```python
from build123d import *

# Parameters (mm, degrees)
EXTRUDE_1_DEPTH     = 15.5
SKETCH_2_R          = 4
CUT_EXTRUDE_1_DEPTH = 41.118574252
SKETCH_3_W          = 25
SKETCH_3_H          = 25.5
CUT_EXTRUDE_2_DEPTH = 43.924352063
CUT_EXTRUDE_3_REACH = 39.346
SKETCH_4_R          = 5.3
FILLET_1_R          = 1
FILLET_2_R          = 1
CHAMFER_1_SIZE      = 0.2


with BuildPart() as part:
    # ｽｹｯﾁ1 → ﾎﾞｽ - 押し出し1 (new, symmetric)
    with BuildSketch(Plane.XY):
        with BuildLine():
            Line((-18.5, 11), (-18.5, -13))
            Line((-18.5, -13), (-11.715374514, -13))
            ThreePointArc((-11.715374514, -13), (12.037359531, -12.702439747), (13.610657589, 11))
            Line((13.610657589, 11), (-18.5, 11))
        make_face()
    extrude(amount=EXTRUDE_1_DEPTH, both=True)

    # ｽｹｯﾁ2 → ｶｯﾄ - 押し出し1 (cut, through all)
    with BuildSketch(Plane.XY.offset(15.5)):
        Circle(SKETCH_2_R)
        with BuildLine():
            Line((-18.5, 2), (-14.5, 2))
            ThreePointArc((-14.5, 2), (-10.5, -2), (-14.5, -6))
            Line((-14.5, -6), (-18.5, -6))
            Line((-18.5, -6), (-18.5, 2))
        make_face()
    extrude(amount=-CUT_EXTRUDE_1_DEPTH, mode=Mode.SUBTRACT)

    # ｽｹｯﾁ3 → ｶｯﾄ - 押し出し2 (cut, through all)
    with BuildSketch(Plane.ZY.offset(18.5)):
        with Locations((0, -4.75)):
            Rectangle(SKETCH_3_W, SKETCH_3_H)
    extrude(amount=-CUT_EXTRUDE_2_DEPTH, mode=Mode.SUBTRACT)

    # ｽｹｯﾁ4 → ｶｯﾄ - 押し出し3 (cut, up to next)
    with BuildSketch(Plane(origin=(0, 11, 0), x_dir=(1, 0, 0), z_dir=(0, 1, 0)), mode=Mode.PRIVATE) as cut_extrude_3_sk1:
        with Locations(Location((1.5, 0, 0), (0, 0, 270))):
            Circle(SKETCH_4_R)
    cut_extrude_3_tool1 = extrude(cut_extrude_3_sk1.sketch, amount=-CUT_EXTRUDE_3_REACH, mode=Mode.PRIVATE) & part.part
    add(cut_extrude_3_tool1.solids().sort_by_distance((1.5, 11, 0))[0], mode=Mode.SUBTRACT)

    # ﾌｨﾚｯﾄ1
    fillet_1_edges = [part.edges().sort_by_distance(p)[0] for p in [
        (-18.5, -6, -14),
        (-18.5, 2, -14),
        (-18.5, -6, 14),
        (-18.5, 2, 14),
        (-18.5, -13, -14),
        (-18.5, -13, 14),
    ]]
    fillet(fillet_1_edges, radius=FILLET_1_R)

    # ﾌｨﾚｯﾄ2
    fillet_2_edges = [part.edges().sort_by_distance(p)[0] for p in [
        (-2.444671206, 11, 15.5),
        (-1.467808792, 8, -12.5),
        (-1.467808792, 8, 12.5),
        (-2.444671206, 11, -15.5),
    ]]
    fillet(fillet_2_edges, radius=FILLET_2_R)

    # 面取り1
    chamfer_1_edges = [part.edges().sort_by_distance(p)[0] for p in [
        (-4, 0, -15.5),
        (-4, 0, 15.5),
        (-4, 0, -12.5),
        (-4, 0, 12.5),
        (1.5, 11, -5.3),
        (1.5, 8, -5.3),
    ]]
    chamfer(chamfer_1_edges, length=CHAMFER_1_SIZE)


solid = part.part
```
Model file for the job. Use its own axes, mm. A direction names the side the tool comes from. Give positions to 0.01 mm unless a question says otherwise; leave off trailing zeros. Loops run counter-clockwise (first coordinate to the right, second up) from the corner with the lowest first, then second, coordinate; pieces in that order, holes last. Notation, with made-up numbers: (86, 37.25) - (114, 37.25) arc R31 cw to (114, 68.25) - close; hole circle Ø4 at (32.5, 4.5). An arc over 180 degrees is marked (long way). One line per item, written item: value. Start each with the question number.
1. Slice it at A-A (z = 0). List the corners of the cut face in (x, y), plus the area to 3 significant figures.
2. Slice it at C-C (x = -13). List the corners of the cut face in (y, z), plus the area to 3 significant figures.
3. Probe L1, parallel to Y at x = 0, z = 13; L2, parallel to Z at x = 5, y = 1.25; L3, parallel to Y at x = 3, z = -13. List the from-to ranges inside material, lowest first. Write a range as from..to.
4. Pin check, flat tips, straight feed: pin 1 (13 mm diameter, centred on x = 0, y = 0, fed in from -Z); pin 2 (10 mm diameter, centred on x = 6, z = -4.5, fed in from -Y); pin 3 (1.5 mm diameter, centred on x = -15.5, z = 14.5, fed in from -Y). Stop position of each tip, or through.
5. Pull direction X, two halves, no side cores. Call faces 1 (the flat face through (-16, 2, 14)), 2 (the flat face through (-18.5, -9, -14)), 3 (the cylindrical face through (5.08, 9.52, -3.91)): pulls with the +X half, pulls with the -X half, needs draft (parallel to the pull), parting line crosses it, or undercut.
6. Slice it at B-B (y = 0). List the corners of the cut face in (x, z), plus the area to 3 significant figures.
7. Which spindle directions (+Z, -Z, +X, -X, +Y, -Y) get a long thin tool onto all of the face, cutting with end or side? Do faces 4 (the cylindrical face through (-0.989, 7.715, -12.199)), 5 (the flat face through (-1, -7, -15.5)), 6 (the cylindrical face through (-18.215, -6.301, 13.979)), 7 (the cylindrical face through (-2.299, 10.715, -15.199)), 8 (the flat face through (-15, -13, 14)). Say none if no direction does.
8. Slice it at D-D (y = 9). List the corners of the cut face in (x, z).
Solution:
1. outline: (-18.5, 8) - (-4, 8) - (-3.8, 8.2) - (-3.8, 10.8) - (-4, 11) - (-18.5, 11) - close; (6.8, 8.2) - (7, 8) - (15.56, 8) arc R17.5 ccw to (13.61, 11) - (7, 11) - (6.8, 10.8) - close
1. area: 67.6 mm^2
2. outline: (-13, -15.5) - (-5.71, -15.5) - (-5.71, -12.5) - (-13, -12.5) - close; (-13, 12.5) - (-5.71, 12.5) - (-5.71, 15.5) - (-13, 15.5) - close; (1.71, -15.5) - (10, -15.5) arc R1 ccw to (11, -14.5) - (11, 14.5) arc R1 ccw to (10, 15.5) - (1.71, 15.5) - (1.71, 12.5) - (7, 12.5) arc R1 cw to (8, 11.5) - (8, -11.5) arc R1 cw to (7, -12.5) - (1.71, -12.5) - close
2. area: 175 mm^2
3. L1: y = -17.5..-4, 4..11
3. L2: z = -15.5..-12.5, 12.5..15.5
3. L3: y = -17.24..-2.65, 2.65..11
4. pin 1: stops at z = -15.5
4. pin 2: stops at y = 8
4. pin 3: stops at y = -13
5. face 1: needs draft
5. face 2: pulls with the -X half
5. face 3: undercut
6. outline: (-11.04, -15.5) - (-4.2, -15.5) - (-4, -15.3) - (-4, -12.7) - (-4.2, -12.5) - (-11.04, -12.5) - close; (-11.04, 12.5) - (-4.2, 12.5) - (-4, 12.7) - (-4, 15.3) - (-4.2, 15.5) - (-11.04, 15.5) - close; (4, -15.3) - (4.2, -15.5) - (17.5, -15.5) - (17.5, -12.5) - (4.2, -12.5) - (4, -12.7) - close; (4, 12.7) - (4.2, 12.5) - (17.5, 12.5) - (17.5, 15.5) - (4.2, 15.5) - (4, 15.3) - close
6. area: 123 mm^2
7. face 4: +X, -X, -Y
7. face 5: -Z, +X, -X, +Y, -Y
7. face 6: +Z, -Z, -X
7. face 7: -Z, +X, -X, +Y
7. face 8: +Z, -Z, -X, -Y
8. outline: (-18.5, -15.5) - (15.01, -15.5) - (15.01, 15.5) - (-18.5, 15.5) - close; hole circle Ø10.6 at (1.5, 0)
